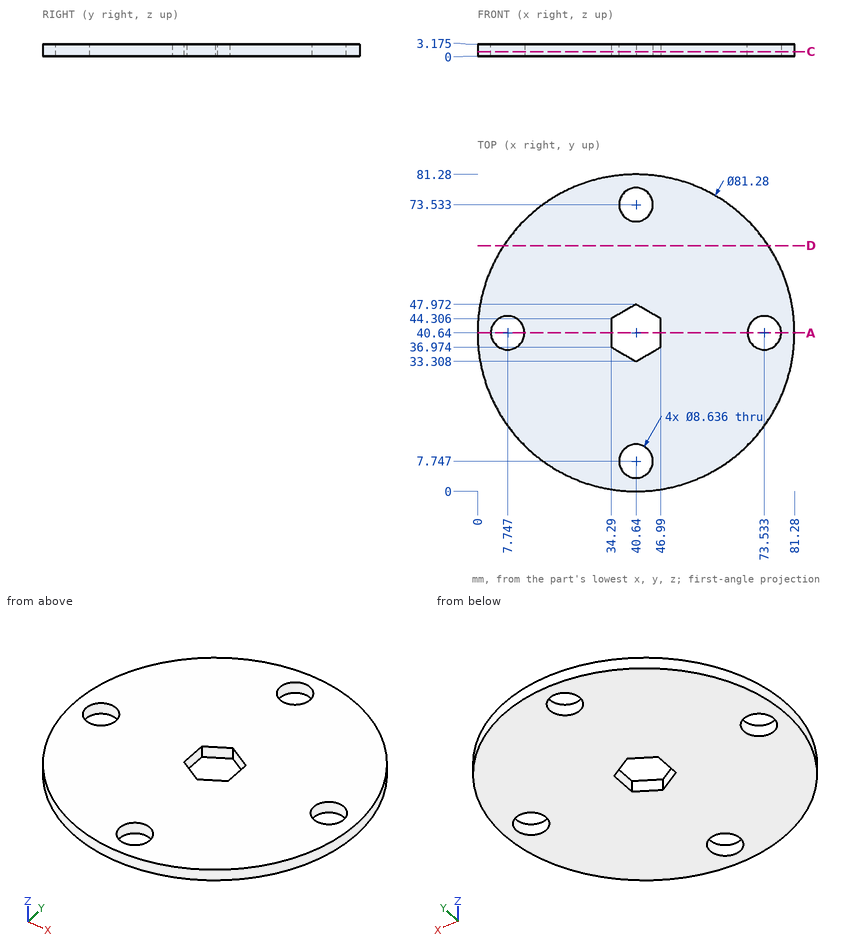
Geometry check sheet. Reference: drawing and pictorial views, mm from the part's lowest x, y, z. Give positions to 0.01 mm unless a question says otherwise; leave off trailing zeros. Order: outer loops, then holes, each group sorted by start corner. A loop starts at its lowest first (then second) coordinate and runs counter-clockwise, first axis right, second up. Notation, with made-up numbers: M 85.5,-15 L 103.5,-15 A18 cw 103.5,17 Z; hole C -8.5,80 d4. An arc over 180 degrees is marked long. Answer as a JSON object with one key per item and string values. Group by question number.
1) Scan lines: line 1 along Y through (x, z) = (37, 1.05) (1 decimal); line 2 along Y through (x, z) = (72, 0.55) (1 decimal); line 3 along X through (y, z) = (8.5, 2.45). Record each from-to range of solid material in increasing order. Write a range as [from, to].
2) Cross-section at D-D (y = 63). Enter the section's corners in (x, z) (1 decimal).
3) Depth check by flat-ended pin: pin 1 Ø1 at (x, z) = (45, 2) entering from -Y; pin 2 Ø1 at (y, z) = (53.5, 2) entering from -X (1 decimal). Enter the tip coordinate at first touch or a pass-through.
4) Cross-section at A-A (y = 40.64). Enter the section's corners in (x, z) (1 decimal), then the cut area to 3 significant figures.
5) Cross-section at C-C (z = 1.2). Enter the section's corners in (x, y) (1 decimal), then the cut area to 3 significant figures.
Result sheet:
{
 "1": {"line 1": "y = [0.2, 5.4], [10.1, 35.4], [45.9, 71.2], [75.9, 81.1]", "line 2": "y = [14.8, 36.6], [44.7, 66.5]", "line 3": "x = [15.77, 36.39], [44.89, 65.51]"},
 "2": {"outline": "M 6.7,0 L 74.6,0 L 74.6,3.2 L 6.7,3.2 Z"},
 "3": {"pin 1": "stops at y = 0.18", "pin 2": "stops at x = 1.9"},
 "4": {"outline": "M 0,0 L 3.4,0 L 3.4,3.2 L 0,3.2 Z; M 12.1,0 L 34.3,0 L 34.3,3.2 L 12.1,3.2 Z; M 47,0 L 69.2,0 L 69.2,3.2 L 47,3.2 Z; M 77.9,0 L 81.3,0 L 81.3,3.2 L 77.9,3.2 Z", "area": "163 mm2"},
 "5": {"outline": "C 40.6,40.6 d81.3; hole C 7.7,40.6 d8.6; hole M 34.3,37 L 40.6,33.3 L 47,37 L 47,44.3 L 40.6,48 L 34.3,44.3 Z; hole C 40.6,7.7 d8.6; hole C 40.6,73.5 d8.6; hole C 73.5,40.6 d8.6", "area": "4,810 mm2"}
}
